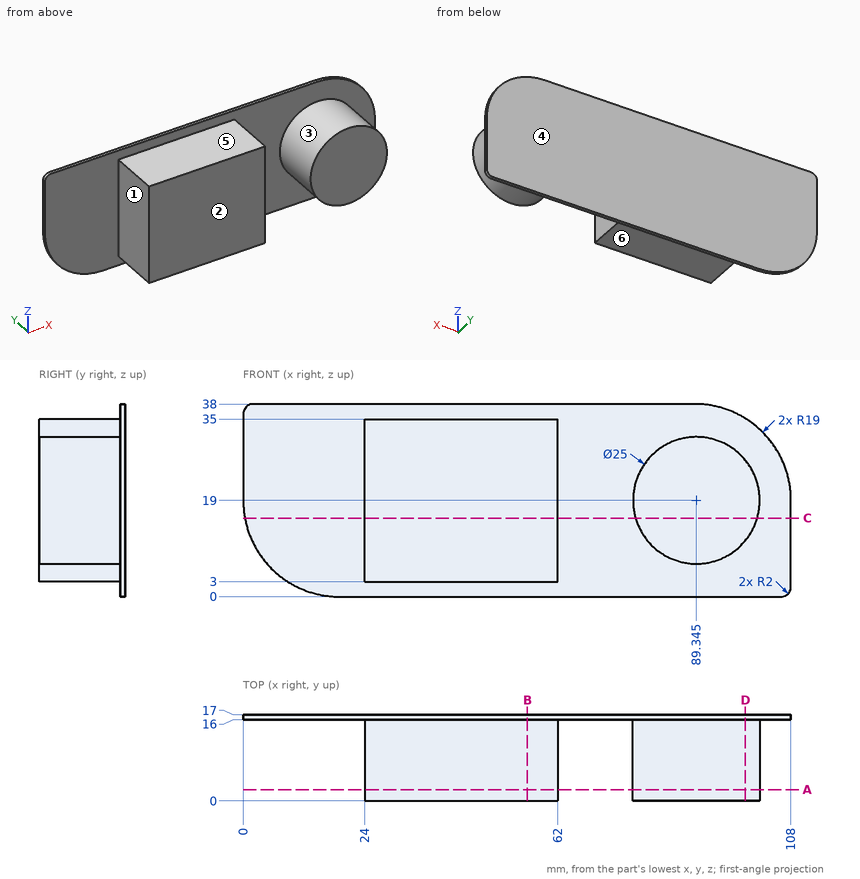
Answer from the drawing. Dimensions are ordinates in mm from the lowest x, y and z of the part. A direction names the side the tool comes from. Give positions to 0.01 mm unless a question says otherwise; leave off trailing zeros. Loops run counter-clockwise (first coordinate to the right, second up) from the corner with the lowest first, then second, coordinate; pieces in that order, holes last. Notation, with made-up numbers: (32, 45.5) - (83, 45.5) arc R6 ccw to (83, 51.5) - close; hole circle Ø2 at (-15.5, -38). An arc over 180 degrees is marked (long way). Answer as a JSON object with one key per item and string values.
1. A cutting plane is placed at B-B (x = 56). Write down the section's boundary in (y, z), then the cut area to 3 significant figures.
Determined:
{"outline": "(0, 3) - (16, 3) - (16, 0) - (17, 0) - (17, 38) - (16, 38) - (16, 35) - (0, 35) - close", "area": "550 mm²"}
2. For the marked faces 4, 5 and 6, determine the directions among +Z, -Z, +X, -X, +Y, -Y from which every point of the face is accessible in a straight line to the end or side of a thin tool.
Determined:
{"face 4": "+Z, -Z, +X, -X, +Y", "face 5": "+Z, +X, -X, -Y", "face 6": "-Z, +X, -X, -Y"}
3. A cutting plane is placed at C-C (z = 15.5). Write down the section's boundary in (x, y) (3 decimals), then the cut area to 3 significant figures.
Determined:
{"outline": "(0.325, 16) - (24, 16) - (24, 0) - (62, 0) - (62, 16) - (77.345, 16) - (77.345, 0) - (101.345, 0) - (101.345, 16) - (108, 16) - (108, 17) - (0.325, 17) - close", "area": "1,100 mm²"}
4. A cutting plane is placed at A-A (y = 2.25). Write down the section's boundary in (x, z) (3 decimals).
Determined:
{"outline": "(24, 3) - (62, 3) - (62, 35) - (24, 35) - close; circle Ø25 at (89.345, 19)"}
5. Flat-ended cylindrical pins translate along their axes: pin 1 Ø8 at (y, z) = (5, 23.5) entering from -X; pin 2 Ø2 at (y, z) = (2.5, 17.5) entering from +X (3 decimals); pin 3 Ø5 at (x, y) = (44.5, 11) entering from +Z; pin 4 Ø8 at (x, y) = (52, 12.5) entering from -Z. Find the tip coordinate at first contact, or state that the pin passes through.
Determined:
{"pin 1": "x = 24", "pin 2": "x = 101.835", "pin 3": "z = 35", "pin 4": "z = 0"}
6. A cutting plane is placed at D-D (x = 99). Write down the section's boundary in (y, z), then the cut area to 3 significant figures.
Determined:
{"outline": "(0, 11.06) - (16, 11.06) - (16, 0) - (17, 0) - (17, 35.16) - (16, 35.16) - (16, 26.94) - (0, 26.94) - close", "area": "289 mm²"}
7. For a pull along X with two mould halves and no side action, classify the marked faces 1, 2 and 3 as pulls with the +X half, pulls with the -X half, needs draft (parallel to the pull), parting line crosses it, or undercut.
Determined:
{"face 1": "pulls with the -X half", "face 2": "needs draft", "face 3": "undercut"}
8. Find the intervals of material crossed by L1, parallel to Y at x = 41, z = 36.5; L2, parallel to X at y = 8, z = 13; L3, parallel to Z at x = 56.5, y = 15, in increasing order. Write a range as [from, to].
Determined:
{"L1": "[16, 17]", "L2": "[24, 62], [78.38, 100.31]", "L3": "[3, 35]"}
